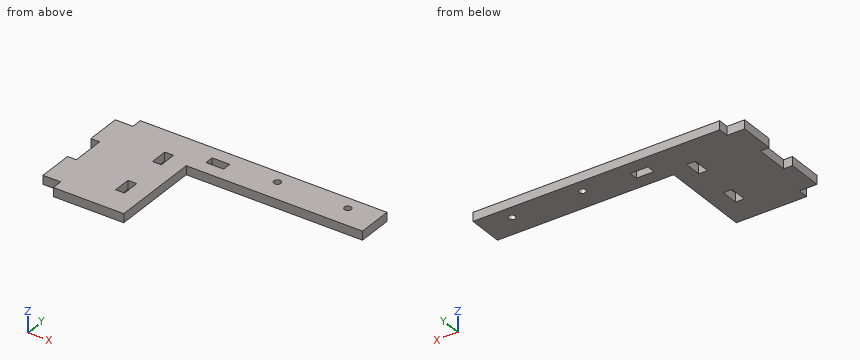
Autodesk Inventor part; units mm, degrees
ref_plane "YZ Plane" through (0, 0, 0) normal (1, 0, 0) x (0, 1, 0)
ref_plane "XZ Plane" through (0, 0, 0) normal (0, 1, 0) x (-1, 0, 0)
ref_plane "XY Plane" through (0, 0, 0) normal (0, 0, 1) x (1, 0, 0)
sketch "Sketch2" plane through (0, 0, 0) normal (0, 0, 1) x (1, 0, 0)
  line L0 (-75.3899, 25.3495) -> (108.7601, 25.3495)
  line L1 (108.7601, 25.3495) -> (108.7601, -0.0505)
  line L2 (108.7601, -0.0505) -> (-18.2399, -0.0505)
  line L3 (-75.3899, 25.3495) -> (-75.3899, -64.8205)
  line L4 (-75.3899, -64.8205) -> (-18.2399, -64.8205)
  line L5 (-18.2399, -64.8205) -> (-18.2399, -0.0505)
  line L6 (-75.3899, 25.3495) -> (-81.7399, 25.3495)
  line L7 (-81.7399, 25.3495) -> (-81.7399, -0.0505)
  line L8 (-81.7399, -0.0505) -> (-75.3899, -0.0505)
  line L9 (-75.3899, -64.8205) -> (-81.7399, -64.8205)
  line L10 (-81.7399, -64.8205) -> (-81.7399, -39.4205)
  line L11 (-81.7399, -39.4205) -> (-75.3899, -39.4205)
  line L12 (108.7601, 25.3495) -> (87.1701, 25.3495)
  line L13 (87.1701, 25.3495) -> (87.1701, 15.8245)
  line L14 (87.1701, 15.8245) -> (36.3701, 15.8245)
  circle A0 centre (36.3701, 15.8245) radius 2.4892
  circle A1 centre (87.1701, 15.8245) radius 2.4892
  line L15 (-18.2399, -64.8205) -> (-18.2399, -45.7705)
  line L16 (-18.2399, -45.7705) -> (-37.2899, -45.7705)
  line L17 (-37.2899, -45.7705) -> (-37.2899, -33.0705)
  line L18 (-37.2899, -33.0705) -> (-30.9399, -33.0705)
  line L19 (-30.9399, -33.0705) -> (-30.9399, -7.6705)
  line L20 (-30.9399, -7.6705) -> (-37.2899, -7.6705)
  line L21 (-37.2899, -7.6705) -> (-37.2899, 5.0295)
  line L22 (-37.2899, 5.0295) -> (-30.9399, 5.0295)
  line L23 (-30.9399, 5.0295) -> (-30.9399, -7.6705)
  line L24 (-30.9399, -33.0705) -> (-30.9399, -45.7705)
  point P0 (0, 0)
  dimension "d5" = 184.15
  dimension "d6" = 25.4
  dimension "d7" = 127
  dimension "d8" = 90.17
  dimension "d9" = 6.35
  dimension "d10" = 25.4
  dimension "d11" = 25.4
  dimension "d12" = 21.59
  dimension "d13" = 9.525
  dimension "d14" = 50.8
  dimension "d15" = 4.9784
  dimension "d16" = 4.9784
  dimension "d17" = 19.05
  dimension "d18" = 19.05
  dimension "d19" = 12.7
  dimension "d20" = 6.35
  dimension "d21" = 25.4
  dimension "d22" = 6.35
  dimension "d23" = 12.7
extrude "Extrusion1" add sketch "Sketch2" along normal blind 6.35
sketch "Sketch3" plane through (0, 0, 6.35) normal (0, 0, 1) x (1, 0, 0)
  line L0 (-81.7399, 25.3495) -> (108.7601, 25.3495)
  line L1 (-81.7399, -0.0505) -> (-81.7399, 25.3495)
  line L2 (-75.3899, -0.0505) -> (-81.7399, -0.0505)
  line L3 (-81.7399, -39.4205) -> (-75.3899, -39.4205)
  line L4 (-81.7399, -64.8205) -> (-81.7399, -39.4205)
  line L5 (-18.2399, -64.8205) -> (-81.7399, -64.8205)
  line L6 (-75.3899, -0.0505) -> (-75.3899, 12.6495)
  line L7 (-75.3899, 12.6495) -> (-69.0399, 12.6495)
  line L8 (-69.0399, 12.6495) -> (-69.0399, 25.3495)
  line L9 (-75.3899, -39.4205) -> (-75.3899, -52.1205)
  line L10 (-75.3899, -52.1205) -> (-69.0399, -52.1205)
  line L11 (-69.0399, -52.1205) -> (-69.0399, -64.8205)
  point P0 (0, 0)
  dimension "d26" = 12.7
  dimension "d27" = 6.35
  dimension "d28" = 12.7
  dimension "d29" = 6.35
extrude "Extrusion2" cut sketch "Sketch3" against normal blind 25.4
sketch "Sketch4" plane through (0, 0, 6.35) normal (0, 0, 1) x (1, 0, 0)
  line L0 (-75.3899, 12.6495) -> (-75.3899, -52.1205)
  line L1 (-75.3899, -52.1205) -> (-69.0399, -52.1205)
  line L2 (-69.0399, -52.1205) -> (-69.0399, -64.8205)
  line L3 (-69.0399, 25.3495) -> (-69.0399, 12.6495)
  line L4 (-69.0399, 12.6495) -> (-75.3899, 12.6495)
  line L5 (-69.0399, 25.3495) -> (-69.0399, 17.7295)
  line L6 (-69.0399, 17.7295) -> (-81.7399, 17.7295)
  line L7 (-81.7399, 17.7295) -> (-81.7399, -7.6705)
  line L8 (-81.7399, -7.6705) -> (-75.3899, -7.6705)
  line L9 (-69.0399, -64.8205) -> (-69.0399, -57.2005)
  line L10 (-69.0399, -57.2005) -> (-81.7399, -57.2005)
  line L11 (-81.7399, -57.2005) -> (-81.7399, -31.8005)
  line L12 (-81.7399, -31.8005) -> (-75.3899, -31.8005)
  point P0 (0, 0)
  dimension "d32" = 7.62
  dimension "d33" = 12.7
  dimension "d34" = 25.4
  dimension "d35" = 7.62
  dimension "d36" = 12.7
  dimension "d37" = 25.4
extrude "Extrusion3" add sketch "Sketch4" against normal blind 25.4
sketch "Sketch5" plane through (0, 0, 6.35) normal (0, 0, 1) x (1, 0, 0)
  line L0 (-81.7399, -57.2005) -> (-69.0399, -57.2005)
  line L1 (-69.0399, 17.7295) -> (-81.7399, 17.7295)
  line L2 (-30.9399, -33.0705) -> (-30.9399, -45.7705)
  line L3 (-69.0399, 17.7295) -> (-69.0399, 15.1895)
  line L4 (-69.0399, 15.1895) -> (-75.3899, 15.1895)
  line L5 (-75.3899, 15.1895) -> (-75.3899, 17.7295)
  line L6 (-69.0399, -57.2005) -> (-69.0399, -54.6605)
  line L7 (-69.0399, -54.6605) -> (-75.3899, -54.6605)
  line L8 (-75.3899, -54.6605) -> (-75.3899, -57.2005)
  point P0 (0, 0)
  dimension "d40" = 2.54
  dimension "d41" = 2.54
extrude "Extrusion4" cut sketch "Sketch5" against normal blind 25.4
sketch "Sketch6" plane through (-81.7399, -7.6705, 6.35) normal (-1, 0, 0) x (0, 0, 1)
  line L0 (0, 25.4) -> (-25.4, 25.4)
  line L1 (0, 25.4) -> (-6.35, 25.4)
  line L2 (-6.35, 25.4) -> (-6.35, -76.2)
  line L3 (-6.35, -76.2) -> (-39.1891, -38.2837)
  line L4 (-39.1891, -38.2837) -> (-39.1891, 49.1671)
  line L5 (-39.1891, 49.1671) -> (-6.35, 49.1671)
  line L6 (-6.35, 49.1671) -> (-6.35, 25.4)
  point P0 (-6.35, 7.6705)
  dimension "d44" = 101.6
extrude "Extrusion5" cut sketch "Sketch6" against normal blind 25.4
sketch "Sketch7" plane through (0, 0, 6.35) normal (0, 0, 1) x (1, 0, 0)
  line L0 (-75.3899, 15.1895) -> (-75.3899, 17.7295)
  line L1 (-75.3899, -57.2005) -> (-75.3899, -54.6605)
  line L2 (-75.3899, -54.6605) -> (-69.0399, -54.6605)
  line L3 (-69.0399, -54.6605) -> (-69.0399, -64.8205)
  line L4 (-69.0399, 25.3495) -> (-69.0399, 15.1895)
  line L5 (-69.0399, 15.1895) -> (-75.3899, 15.1895)
  line L6 (-75.3899, 17.7295) -> (-69.0399, 17.7295)
  line L7 (-75.3899, -57.2005) -> (-69.0399, -57.2005)
  point P0 (0, 0)
extrude "Extrusion6" add sketch "Sketch7" against normal blind 6.35
sketch "Sketch8" plane through (0, 0, 6.35) normal (0, 0, 1) x (1, 0, 0)
  line L0 (108.7601, -0.0505) -> (-18.2399, -0.0505)
  line L1 (-69.0399, 25.3495) -> (108.7601, 25.3495)
  line L2 (108.7601, 25.3495) -> (14.7801, 25.3495)
  line L3 (14.7801, 25.3495) -> (14.7801, 9.4745)
  line L4 (14.7801, 9.4745) -> (14.7801, 15.8245)
  line L5 (14.7801, 15.8245) -> (2.0801, 15.8245)
  line L6 (2.0801, 15.8245) -> (2.0801, 9.4745)
  line L7 (2.0801, 9.4745) -> (-10.6199, 9.4745)
  line L8 (-10.6199, 9.4745) -> (-10.6199, 15.8245)
  line L9 (-10.6199, 15.8245) -> (2.0801, 15.8245)
  point P0 (0, 0)
  dimension "d49" = 93.98
  dimension "d50" = 15.875
  dimension "d51" = 6.35
  dimension "d52" = 12.7
  dimension "d53" = 12.7
extrude "Extrusion7" cut sketch "Sketch8" against normal blind 25.4
properties part number "side 2"
The model under review builds one solid part; all positions refer to its coordinate system, in mm. Round coordinates to 2 decimals unless told otherwise and drop trailing zeros. Order: outer loops, then holes, each group sorted by start corner. A loop starts at its lowest first (then second) coordinate and runs counter-clockwise, first axis right, second up. Notation, with made-up numbers: M 3.25,70 L 56.25,70 A12 cw 56.25,81 Z; hole C 45.25,6.25 d10. An arc over 180 degrees is marked long. Use a Markdown table: item, result.
1) Insertion check: pin 1 (3 mm diameter, centred on x = 17.5, z = 1, fed in from -Y); pin 2 (1.9 mm diameter, centred on x = -77, z = 4, fed in from +Y); pin 3 (4 mm diameter, centred on x = 87.17, y = 15.82, fed in from -Z); pin 4 (2 mm diameter, centred on y = -10.5, z = 3, fed in from +X). Each pin has a flat end and moves straight along its axis. Give the tip position at first contact, or say it passes through.
Report:
| item | result |
|---|---|
| pin 1 | y = -0.05 |
| pin 2 | y = 17.73 |
| pin 3 | through |
| pin 4 | x = -18.24 |
2) Wall thickness on line 1 along X through (y, z) = (3, 6); line 2 along X through (y, z) = (-37.5, 0.75); line 3 along X through (y, z) = (14.5, 6): over which ranges is each line inside the solid? List them lowest first. Write a range as [from, to].
Report:
| item | result |
|---|---|
| line 1 | [-81.74, -37.29], [-30.94, 108.76] |
| line 2 | [-81.74, -37.29], [-30.94, -18.24] |
| line 3 | [-81.74, -10.62], [2.08, 34.26], [38.48, 85.06], [89.28, 108.76] |
3) Consider section A-A (z = 1.75). Write out the cut boundary in (x, y), then the cut area to 3 significant figures.
Report:
| item | result |
|---|---|
| outline | M -81.74,-57.2 L -69.04,-57.2 L -69.04,-64.82 L -18.24,-64.82 L -18.24,-0.05 L 108.76,-0.05 L 108.76,25.35 L -69.04,25.35 L -69.04,17.73 L -81.74,17.73 L -81.74,-7.67 L -75.39,-7.67 L -75.39,-31.8 L -81.74,-31.8 Z; hole M -37.29,-45.77 L -30.94,-45.77 L -30.94,-33.07 L -37.29,-33.07 Z; hole M -37.29,-7.67 L -30.94,-7.67 L -30.94,5.03 L -37.29,5.03 Z; hole M -10.62,9.47 L 2.08,9.47 L 2.08,15.82 L -10.62,15.82 Z; hole C 36.37,15.82 d4.98; hole C 87.17,15.82 d4.98 |
| area | 8,320 mm^2 |
4) Consider section C-C (x = 19.5). Write out the cut boundary in (y, z).
Report:
| item | result |
|---|---|
| outline | M -0.05,0 L 25.35,0 L 25.35,6.35 L -0.05,6.35 Z |
5) Consider section B-B (y = -44). Write out the cut boundary in (x, z), then the cut area to 3 significant figures.
Report:
| item | result |
|---|---|
| outline | M -81.74,0 L -37.29,0 L -37.29,6.35 L -81.74,6.35 Z; M -30.94,0 L -18.24,0 L -18.24,6.35 L -30.94,6.35 Z |
| area | 363 mm^2 |
